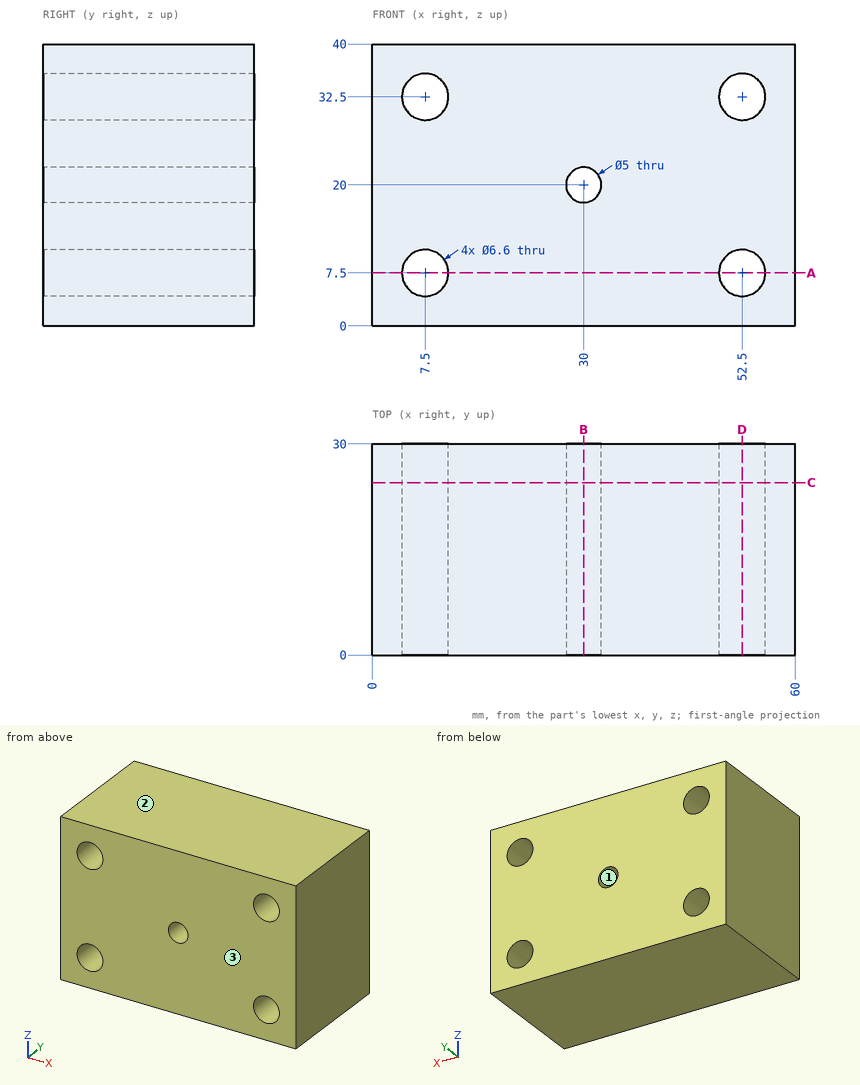
The figure shows three views and two pictorial views of one solid part (mm, origin at its lowest corner). Answer the questions. Give positions to 0.01 mm unless a question says otherwise; leave off trailing zeros. Loops run counter-clockwise (first coordinate to the right, second up) from the corner with the lowest first, then second, coordinate; pieces in that order, holes last. Notation, with made-up numbers: M -35.75,38.25 L -18.75,38.25 A25 ccw -18.75,66.25 Z; hole C 21,48 d9. An arc over 180 degrees is marked long. Write each question's results on one line, items separated by ' | '.
1. The mould has two halves that part along Z. Classify the marked faces 1, 2 and 3: pulls with the +Z half, pulls with the -Z half, needs draft (parallel to the pull), parting line crosses it, or undercut.
Values:
face 1: undercut | face 2: pulls with the +Z half | face 3: needs draft
2. Section D-D on x = 52.5 is taken. Give the vertices of the cut face in (y, z), plus the area to 3 significant figures.
Values:
outline: M 0,0 L 30,0 L 30,4.2 L 0,4.2 Z; M 0,10.8 L 30,10.8 L 30,29.2 L 0,29.2 Z; M 0,35.8 L 30,35.8 L 30,40 L 0,40 Z | area: 804 mm^2
3. Straight lines are drawn through the part: line 1 (Z direction, x = 52.5, y = 8.5); line 2 (Z direction, x = 30, y = 19.25); line 3 (X direction, y = 10, z = 31.5). For each, find the intervals that lie inside material, in ascending order. Write a range as [from, to].
Values:
line 1: z = [0, 4.2], [10.8, 29.2], [35.8, 40] | line 2: z = [0, 17.5], [22.5, 40] | line 3: x = [0, 4.36], [10.64, 49.36], [55.64, 60]
4. Section A-A on z = 7.5 is taken. Give the vertices of the cut face in (x, y), plus the area to 3 significant figures.
Values:
outline: M 0,0 L 4.2,0 L 4.2,30 L 0,30 Z; M 10.8,0 L 49.2,0 L 49.2,30 L 10.8,30 Z; M 55.8,0 L 60,0 L 60,30 L 55.8,30 Z | area: 1,400 mm^2
5. Section B-B on x = 30 is taken. Give the vertices of the cut face in (y, z).
Values:
outline: M 0,0 L 30,0 L 30,17.5 L 0,17.5 Z; M 0,22.5 L 30,22.5 L 30,40 L 0,40 Z
6. Section C-C on y = 24.5 is taken. Give the vertices of the cut face in (x, z).
Values:
outline: M 0,0 L 60,0 L 60,40 L 0,40 Z; hole C 7.5,7.5 d6.6; hole C 7.5,32.5 d6.6; hole C 30,20 d5; hole C 52.5,7.5 d6.6; hole C 52.5,32.5 d6.6
7. Given pin 1 (4 mm diameter, centred on x = 7.5, z = 7.5, fed in from -Y), flat-ended and moving along its own axis, determine where the tip first touches the part or whether it passes through.
Values:
pin 1: passes through
